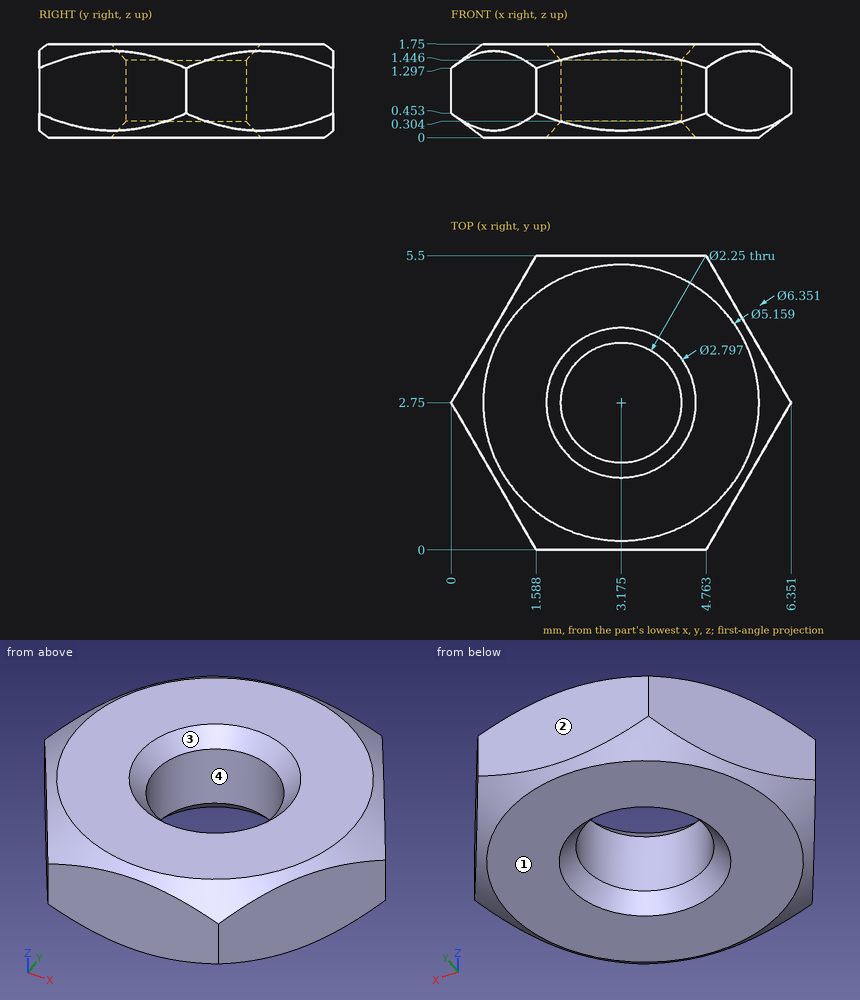
Input: dimensioned drawing with shaded views. Units: mm. Origin: part minimum x, y, z. Round coordinates to 2 decimals unless told otherwise and drop trailing zeros. Use CSV: the item, a comma, the result in double quotes. Start each with the question number.
Q1. Pull-direction query (Y, two-part tool) for the marked faces 1, 2, 3 and 4; classes: pulls with the +Y half, pulls with the -Y half, needs draft (parallel to the pull), parting line crosses it, or undercut.
Q2. First-contact query: pin 1 Ø1 at (y, z) = (3.5, 1.5) entering from +X; pin 2 Ø2.5 at (x, y) = (3.18, 2.75) entering from -Z. Flat tips, straight axial feed; report the tip coordinate or a pass-through.
Q3. Line query: L1, parallel to X at y = 3.4, z = 1.15 (1 decimal); L2, parallel to Y at x = 2.5, z = 0.4; L3, parallel to X at y = 5, z = 0.45. Output: solid intervals per line, ascending.
Result sheet:
1,face 1,"needs draft"
1,face 2,"pulls with the +Y half"
1,face 3,"undercut"
1,face 4,"undercut"
2,pin 1,"x = 6.2"
2,pin 2,"z = 0.16"
3,L1,"0.4 to 2.3, 4.1 to 6"
3,L2,"0 to 1.85, 3.65 to 5.5"
3,L3,"1.3 to 5.05"
